```python
from build123d import *

# Parameters (mm, degrees)
SKETCH1_W               = 60
SKETCH1_H               = 80
SKETCH1_R               = 6.5
BOSS_EXTRUDE4_DEPTH     = 3
BOSS_EXTRUDE5_START     = 30
BOSS_EXTRUDE5_DEPTH     = 15
BOSS_EXTRUDE6_START     = -30
BOSS_EXTRUDE6_DEPTH     = 15
BOSS_EXTRUDE7_DEPTH     = 6
SKETCH1_7_R             = 5.2
CUT_EXTRUDE1_DEPTH      = 7
CUT_EXTRUDE1_DEPTH_BACK = 16


with BuildPart() as part:
    # Sketch1 → Boss-Extrude4 (new body)
    with BuildSketch(Plane(origin=(0, 0, 0), x_dir=(1, 0, 0), z_dir=(0, 1, 0))):
        Rectangle(SKETCH1_W, SKETCH1_H)
        with Locations((5.03, 28.22)):
            Circle(SKETCH1_R, mode=Mode.SUBTRACT)
    extrude(amount=BOSS_EXTRUDE4_DEPTH)

    # Sketch2 → Boss-Extrude5 (add)
    with BuildSketch(Plane(origin=(0, 0, 0), x_dir=(0, 0, -1), z_dir=(1, 0, 0)).offset(BOSS_EXTRUDE5_START)):
        Polygon((-2.920508076, 0), (-11.580762114, 0), (14.4, -15), (29.6, -15), (29.6, -10), (14.4, -10), align=None)
    extrude(amount=-BOSS_EXTRUDE5_DEPTH)

    # Sketch2<3> → Boss-Extrude6 (add)
    with BuildSketch(Plane(origin=(0, 0, 0), x_dir=(0, 0, -1), z_dir=(1, 0, 0)).offset(BOSS_EXTRUDE6_START)):
        Polygon((-2.920508076, 0), (-11.580762114, 0), (14.4, -15), (29.6, -15), (29.6, -10), (14.4, -10), align=None)
    extrude(amount=BOSS_EXTRUDE6_DEPTH)

    # Sketch1<6> → Boss-Extrude7 (add)
    with BuildSketch(Plane(origin=(0, 0, 0), x_dir=(1, 0, 0), z_dir=(0, 1, 0))):
        Polygon((-6.026257655, 28.22), (-0.498128827, 18.645), (10.558128827, 18.645), (16.086257655, 28.22), (10.558128827, 37.795), (-0.498128827, 37.795), align=None)
        Polygon((9.172488181, 35.395), (0.887511819, 35.395), (-3.254976363, 28.22), (0.887511819, 21.045), (9.172488181, 21.045), (13.314976363, 28.22), align=None, mode=Mode.SUBTRACT)
    extrude(amount=BOSS_EXTRUDE7_DEPTH)

    # Sketch1<7> → Cut-Extrude1 (cut, two sides)
    with BuildSketch(Plane(origin=(0, 0, 0), x_dir=(1, 0, 0), z_dir=(0, 1, 0))) as cut_extrude1_sk:
        with Locations((-22.5, 22)):
            Circle(SKETCH1_7_R)
        with Locations((22.5, 22)):
            Circle(SKETCH1_7_R)
    extrude(amount=CUT_EXTRUDE1_DEPTH, mode=Mode.SUBTRACT)
    extrude(cut_extrude1_sk.sketch, amount=-CUT_EXTRUDE1_DEPTH_BACK, mode=Mode.SUBTRACT)


solid = part.part
```
Geometry: final body of the model. Coordinates: model frame, mm. A direction names the side the tool comes from. Give positions to 0.01 mm unless a question says otherwise; leave off trailing zeros. Loops run counter-clockwise (first coordinate to the right, second up) from the corner with the lowest first, then second, coordinate; pieces in that order, holes last. Notation, with made-up numbers: (-37.75, 28) -> (-16.75, 28) arc R16 cw to (-16.75, 53) -> close; hole circle Ø5 at (50.5, 50.25). An arc over 180 degrees is marked (long way). Use CSV: the item, a comma, the result in double quotes.
(1) Cut plane A-A (x = 5.03). Output: boundary loops of the cut face in (y, z) (3 decimals).
From the geometry:
outline,"(0, -40) -> (3, -40) -> (3, -37.795) -> (6, -37.795) -> (6, -35.395) -> (3, -35.395) -> (3, -34.72) -> (0, -34.72) -> close; (0, -21.72) -> (3, -21.72) -> (3, -21.045) -> (6, -21.045) -> (6, -18.645) -> (3, -18.645) -> (3, 40) -> (0, 40) -> close"
(2) Pull-direction query (Z, two-part tool) for faces 6 (the face through (-20.101, -12.465, -17.387)), 7 (the face through (30, -5.4, -5.7)), 8 (the face through (-22.605, -7.395, -1.228)); classes: released by +Z, released by -Z, zero draft, split by the parting line, or undercut.
From the geometry:
face 6,"undercut"
face 7,"zero draft"
face 8,"released by +Z"
(3) First-contact query: P1, Ø21, axis at x = 5.03, z = -28.22, coming from the +Y side; P2, Ø0.9, axis at x = 5, y = 4.5, coming from the +Z side (3 decimals); P3, Ø16.5, axis at x = 23.5, z = -24, coming from the +Y side; P4, Ø5, axis at x = 20, y = -8.5, coming from the +Z side. Flat tips, straight axial feed; report the tip coordinate or a pass-through.
From the geometry:
P1,"y = 6"
P2,"z = -18.645"
P3,"y = 3"
P4,"z = 1.19"
(4) Cut plane C-C (z = 1). Output: boundary loops of the cut face in (x, y), plus the area to 3 significant figures.
From the geometry:
outline,"(-30, -6.11) -> (-15, -6.11) -> (-15, -1.11) -> (-30, -1.11) -> close; (-30, 0) -> (30, 0) -> (30, 3) -> (-30, 3) -> close; (15, -6.11) -> (30, -6.11) -> (30, -1.11) -> (15, -1.11) -> close"
area,"330 mm^2"
(5) Ray query, line 1 along Z through (x, y) = (5.03, 0.6); line 2 along X through (y, z) = (-13.95, -22); line 3 along X through (y, z) = (-11.75, -19.5). Return the intervals inside material, ascending. Write a range as [from, to].
From the geometry:
line 1,"[-40, -34.72], [-21.72, 40]"
line 2,"[-30, -27.7], [-17.3, -15], [15, 17.3], [27.7, 30]"
line 3,"[-30, -27.06], [-17.94, -15], [15, 17.94], [27.06, 30]"
(6) Cut plane D-D (x = 22.5). Output: boundary loops of the cut face in (y, z), plus the area to 3 significant figures.
From the geometry:
outline,"(-15, -29.6) -> (-10, -29.6) -> (-10, -27.2) -> (-15, -27.2) -> close; (-15, -16.8) -> (-10, -16.8) -> (-10, -14.4) -> (0, 2.92) -> (0, -16.8) -> (3, -16.8) -> (3, 40) -> (0, 40) -> (0, 11.58) -> (-15, -14.4) -> close; (0, -40) -> (3, -40) -> (3, -27.2) -> (0, -27.2) -> close"
area,"341 mm^2"
(7) Access query for faces 1 (the face through (-22.6, -5.07, -5.86)), 2 (the face through (11.27, 4.48, -31.76)), 3 (the face through (13.36, 4.48, -32.94)), 4 (the face through (23, -13, -29.6)), 5 (the face through (-15, -9, -10)). Directions: +Z, -Z, +X, -X, +Y, -Y. A direction counts if a zero-diameter tool reaches every point of the face in a straight line with its end or side. Return the directions, or none.
From the geometry:
face 1,"-Z, +X, -X"
face 2,"+Y"
face 3,"-Z, +X, +Y"
face 4,"-Z, +X, -X, -Y"
face 5,"+Z, -Z, -Y"
(8) Cut plane B-B (y = -13.25). Output: boundary loops of the cut face in (x, z).
From the geometry:
outline,"(-30, -29.6) -> (-15, -29.6) -> (-15, -11.37) -> (-30, -11.37) -> close; (15, -29.6) -> (30, -29.6) -> (30, -11.37) -> (15, -11.37) -> close; hole circle Ø10.4 at (-22.5, -22); hole circle Ø10.4 at (22.5, -22)"
